Work out the finished part from the listing and answer in its coordinate system (mm). Give positions to 0.01 mm unless a question says otherwise; leave off trailing zeros. Loops run counter-clockwise (first coordinate to the right, second up) from the corner with the lowest first, then second, coordinate; pieces in that order, holes last. Notation, with made-up numbers: (52, 19.25) -> (111, 19.25) arc R11 ccw to (111, 25.25) -> close; hole circle Ø1 at (10.25, 58). An arc over 180 degrees is marked (long way). Answer as CSV lines item,"result". Start each with the question number.
1. A flat-ended cylindrical pin translates along its axis: pin 1 Ø4 at (x, y) = (31.5, 6) entering from -Z. Find the tip coordinate at first contact, or state that the pin passes through.
2. Find section B-B, the plane z = 25. Give the vertices of the cut face in (x, y).
3. Find section A-A, the plane z = 1. Give the vertices of the cut face in (x, y), and give its area (3 significant figures).
4. Find the intervals of material crossed by line 1 along Z through (x, y) = (-14.5, 3.5); line 2 along Z through (x, y) = (20.5, 4.5); line 3 along Z through (x, y) = (33, 0.5), in increasing order.
5. Find section C-C, the plane y = 6.5. Count the separate pieces of the cut face and the enclosed holes in it, and give its area (3 significant figures).
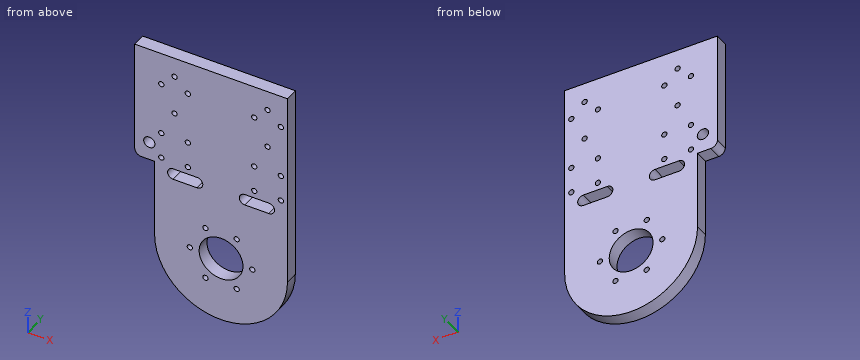
from build123d import *

# Parameters (mm, degrees)
SKETCH1_R           = 16.5
SKETCH1_R_2         = 2
BOSS_EXTRUDE3_DEPTH = 10
SKETCH9_W           = 90
SKETCH9_H           = 10
BOSS_EXTRUDE4_DEPTH = 15
FILLET1_R           = 5
SKETCH10_R          = 4.25
CUT_EXTRUDE7_DEPTH  = 10
CUT_EXTRUDE8_DEPTH  = 10


with BuildPart() as part:
    # Sketch1 → Boss-Extrude3 (new body)
    with BuildSketch(Plane(origin=(0, 0, 0), x_dir=(1, 0, 0), z_dir=(0, 1, 0))):
        with BuildLine():
            Line((-52.326392464, -141.880675109), (47.673607536, -141.880675109))
            Line((47.673607536, -141.880675109), (47.673607536, 8.119324891))
            ThreePointArc((47.673607536, 8.119324891), (-2.326392464, 58.119324891), (-52.326392464, 8.119324891))
            Line((-52.326392464, 8.119324891), (-52.326392464, -141.880675109))
        make_face()
        with Locations((-2.326392464, 8.119324891)):
            Circle(SKETCH1_R, mode=Mode.SUBTRACT)
        with Locations((21.173607536, 8.119324891)):
            Circle(SKETCH1_R_2, mode=Mode.SUBTRACT)
        with Locations((9.423607536, -12.232272098)):
            Circle(SKETCH1_R_2, mode=Mode.SUBTRACT)
        with Locations((-14.076392464, -12.232272098)):
            Circle(SKETCH1_R_2, mode=Mode.SUBTRACT)
        with Locations((-25.826392464, 8.119324891)):
            Circle(SKETCH1_R_2, mode=Mode.SUBTRACT)
        with Locations((-14.076392464, 28.47092188)):
            Circle(SKETCH1_R_2, mode=Mode.SUBTRACT)
        with Locations((9.423607536, 28.47092188)):
            Circle(SKETCH1_R_2, mode=Mode.SUBTRACT)
        with Locations((-47.326392464, -116.880675109)):
            Circle(SKETCH1_R_2, mode=Mode.SUBTRACT)
        with Locations((42.673607536, -116.880675109)):
            Circle(SKETCH1_R_2, mode=Mode.SUBTRACT)
        with Locations((-37.326392464, -126.880675109)):
            Circle(SKETCH1_R_2, mode=Mode.SUBTRACT)
        with Locations((-37.326392464, -96.880675109)):
            Circle(SKETCH1_R_2, mode=Mode.SUBTRACT)
        with Locations((-47.326392464, -76.880675109)):
            Circle(SKETCH1_R_2, mode=Mode.SUBTRACT)
        with Locations((42.673607536, -76.880675109)):
            Circle(SKETCH1_R_2, mode=Mode.SUBTRACT)
        with Locations((-47.326392464, -56.880675109)):
            Circle(SKETCH1_R_2, mode=Mode.SUBTRACT)
        with Locations((42.673607536, -56.880675109)):
            Circle(SKETCH1_R_2, mode=Mode.SUBTRACT)
        with Locations((-27.326392464, -116.880675109)):
            Circle(SKETCH1_R_2, mode=Mode.SUBTRACT)
        with Locations((22.673607536, -116.880675109)):
            Circle(SKETCH1_R_2, mode=Mode.SUBTRACT)
        with Locations((-27.326392464, -56.880675109)):
            Circle(SKETCH1_R_2, mode=Mode.SUBTRACT)
        with Locations((-27.326392464, -76.880675109)):
            Circle(SKETCH1_R_2, mode=Mode.SUBTRACT)
        with Locations((22.673607536, -56.880675109)):
            Circle(SKETCH1_R_2, mode=Mode.SUBTRACT)
        with Locations((22.673607536, -76.880675109)):
            Circle(SKETCH1_R_2, mode=Mode.SUBTRACT)
        with Locations((32.673607536, -96.880675109)):
            Circle(SKETCH1_R_2, mode=Mode.SUBTRACT)
        with Locations((32.673607536, -126.880675109)):
            Circle(SKETCH1_R_2, mode=Mode.SUBTRACT)
    extrude(amount=BOSS_EXTRUDE3_DEPTH)

    # Sketch9 → Boss-Extrude4 (add)
    with BuildSketch(Plane.ZY.offset(52.326392464)):
        with Locations((96.880675109, 5)):
            Rectangle(SKETCH9_W, SKETCH9_H)
    extrude(amount=BOSS_EXTRUDE4_DEPTH)

    # Fillet1
    fillet1_edges = [part.edges().sort_by_distance(p)[0] for p in [
        (-67.326392464, 5, 51.880675109),
    ]]
    fillet(fillet1_edges, radius=FILLET1_R)

    # Sketch10 → Cut-Extrude7 (cut)
    with BuildSketch(Plane(origin=(0, 10, 0), x_dir=(1, 0, 0), z_dir=(0, 1, 0))):
        with Locations((-56.326392464, -65.880675109)):
            Circle(SKETCH10_R)
    extrude(amount=-CUT_EXTRUDE7_DEPTH, mode=Mode.SUBTRACT)

    # Sketch11 → Cut-Extrude8 (cut)
    with BuildSketch(Plane(origin=(0, 10, 0), x_dir=(1, 0, 0), z_dir=(0, 1, 0))):
        with BuildLine():
            Line((15.673607536, -42.630675109), (33.673607536, -42.630675109))
            ThreePointArc((33.673607536, -42.630675109), (37.923607536, -46.880675109), (33.673607536, -51.130675109))
            Line((33.673607536, -51.130675109), (15.673607536, -51.130675109))
            ThreePointArc((15.673607536, -51.130675109), (11.423607536, -46.880675109), (15.673607536, -42.630675109))
        make_face()
        with BuildLine():
            Line((-38.326392464, -42.630675109), (-20.326392464, -42.630675109))
            ThreePointArc((-20.326392464, -42.630675109), (-16.076392464, -46.880675109), (-20.326392464, -51.130675109))
            Line((-20.326392464, -51.130675109), (-38.326392464, -51.130675109))
            ThreePointArc((-38.326392464, -51.130675109), (-42.576392464, -46.880675109), (-38.326392464, -42.630675109))
        make_face()
    extrude(amount=-CUT_EXTRUDE8_DEPTH, mode=Mode.SUBTRACT)


solid = part.part
Resolved:
1,pin 1,"stops at z = -46.68"
2,outline,"(-52.33, 0) -> (47.67, 0) -> (47.67, 10) -> (-52.33, 10) -> close"
3,outline,"(-52.33, 0) -> (-16.08, 0) -> (-16.08, 10) -> (-52.33, 10) -> close; (11.42, 0) -> (47.67, 0) -> (47.67, 10) -> (11.42, 10) -> close"
3,area,"725 mm^2"
4,line 1,"z = -56.61 to -30.43, -26.52 to -19.26, 3.02 to 10.28, 14.19 to 141.88"
4,line 2,"z = -52.6 to -10, -6.24 to 42.63, 51.13 to 141.88"
4,line 3,"z = -43.5 to 42.63, 51.13 to 94.91, 98.85 to 124.91, 128.85 to 141.88"
5,separate pieces,"1"
5,enclosed holes,"26"
5,area,"18,700 mm^2"
